CAD build for the part. Positions are in the model's coordinates, mm. Face numbers are marked on the shaded views. Round coordinates to 2 decimals unless told otherwise and drop trailing zeros. Loops run counter-clockwise (first coordinate to the right, second up) from the corner with the lowest first, then second, coordinate; pieces in that order, holes last. Notation, with made-up numbers: (59.5, 74) -> (113.5, 74) arc R19 cw to (113.5, 86) -> close; hole circle Ø10 at (10, 35). An arc over 180 degrees is marked (long way). Answer as CSV lines item,"result".
```python
from build123d import *

# Parameters (mm, degrees)
BOSS_EXTRUDE1_DEPTH = 600
CUT_EXTRUDE1_DEPTH  = 200
BOSS_EXTRUDE2_DEPTH = 20
FILLET1_R           = 5
SKETCH4_R           = 35
BOSS_EXTRUDE3_DEPTH = 20
BOSS_EXTRUDE4_START = 20
SKETCH5_R           = 35
BOSS_EXTRUDE4_DEPTH = 20
SKETCH6_R           = 10
CUT_EXTRUDE2_DEPTH  = 741.945342114
SKETCH7_R           = 25
BOSS_EXTRUDE5_DEPTH = 60
SKETCH9_R           = 20
CUT_EXTRUDE3_DEPTH  = 749.999332443
SKETCH10_R          = 7.841324839
BOSS_EXTRUDE6_DEPTH = 40
SKETCH11_R          = 3.5
BOSS_EXTRUDE7_DEPTH = 300
SKETCH12_R          = 4.427649499
BOSS_EXTRUDE8_DEPTH = 10


with BuildPart() as part:
    # Sketch1 → Boss-Extrude1 (new body)
    with BuildSketch(Plane.XY):
        Polygon((280, -110), (350, -40), (350, 110), (-350, 110), (-350, -110), align=None)
    extrude(amount=BOSS_EXTRUDE1_DEPTH)

    # Sketch2 → Cut-Extrude1 (cut)
    with BuildSketch(Plane(origin=(0, 110, 0), x_dir=(1, 0, 0), z_dir=(0, 1, 0))):
        Polygon((20.098635598, -30), (90.098635598, -300), (20.098635598, -570), (-320, -570), (-320, -30), align=None)
    extrude(amount=-CUT_EXTRUDE1_DEPTH, mode=Mode.SUBTRACT)

    # Sketch3 → Boss-Extrude2 (add)
    with BuildSketch(Plane(origin=(0, 110, 0), x_dir=(1, 0, 0), z_dir=(0, 1, 0))):
        Polygon((-330, -20), (-330, -580), (27.836654621, -580), (100.429247214, -300), (27.836654621, -20), align=None)
        Polygon((-320, -30), (-320, -570), (20.098635598, -570), (90.098635598, -300), (20.098635598, -30), align=None, mode=Mode.SUBTRACT)
    extrude(amount=BOSS_EXTRUDE2_DEPTH)

    # Fillet1
    fillet1_edges = [part.edges().sort_by_distance(p)[0] for p in [
        (-151.081672689, 130, 20),
        (-330, 130, 300),
        (-151.081672689, 130, 580),
        (64.132950917, 130, 440),
        (64.132950917, 130, 160),
        (-149.950682201, 130, 30),
        (-320, 130, 300),
        (-149.950682201, 130, 570),
        (55.098635598, 130, 435),
        (55.098635598, 130, 165),
    ]]
    fillet(fillet1_edges, radius=FILLET1_R - 0.0001)  # a hair under: the kernel refuses the full size

    # Sketch4 → Boss-Extrude3 (add)
    with BuildSketch(Plane.XY.offset(600)):
        with Locations(Location((270, 40, 0), (0, 0, 180))):
            Circle(SKETCH4_R)
    extrude(amount=BOSS_EXTRUDE3_DEPTH)

    # Sketch5 → Boss-Extrude4 (add)
    with BuildSketch(Plane(origin=(0, 0, 0), x_dir=(-1, 0, 0), z_dir=(0, 0, -1)).offset(BOSS_EXTRUDE4_START)):
        with Locations((-270, 40)):
            Circle(SKETCH5_R)
    extrude(amount=-BOSS_EXTRUDE4_DEPTH)

    # Sketch6 → Cut-Extrude2 (cut, through all)
    with BuildSketch(Plane.XY.offset(620)):
        with Locations((270, 40)):
            Circle(SKETCH6_R)
    extrude(amount=-CUT_EXTRUDE2_DEPTH, mode=Mode.SUBTRACT)

    # Sketch7 → Boss-Extrude5 (add)
    with BuildSketch(Plane(origin=(0, 110, 0), x_dir=(1, 0, 0), z_dir=(0, 1, 0))):
        with Locations(Location((177.752116484, -300, 0), (0, 0, 90))):
            Circle(SKETCH7_R)
    extrude(amount=BOSS_EXTRUDE5_DEPTH)

    # Sketch9 → Cut-Extrude3 (cut, through all)
    with BuildSketch(Plane.XY.offset(620)):
        with Locations((270, 40)):
            Circle(SKETCH9_R)
    extrude(amount=-CUT_EXTRUDE3_DEPTH, mode=Mode.SUBTRACT)

    # Sketch10 → Boss-Extrude6 (add)
    with BuildSketch(Plane(origin=(0, 110, 0), x_dir=(1, 0, 0), z_dir=(0, 1, 0))):
        with Locations(Location((-338.53526131, -590.113534013, 0), (0, 0, 90))):
            Circle(SKETCH10_R)
    extrude(amount=BOSS_EXTRUDE6_DEPTH)

    # Sketch11 → Boss-Extrude7 (add)
    with BuildSketch(Plane(origin=(0, 150, 0), x_dir=(1, 0, 0), z_dir=(0, 1, 0))):
        with Locations(Location((-338.53526131, -590.113534013, 0), (0, 0, 270))):
            Circle(SKETCH11_R)
    extrude(amount=BOSS_EXTRUDE7_DEPTH)

    # Sketch12 → Boss-Extrude8 (add)
    with BuildSketch(Plane(origin=(0, 450, 0), x_dir=(1, 0, 0), z_dir=(0, 1, 0))):
        with Locations(Location((-338.53526131, -590.113534013, 0), (0, 0, 270))):
            Circle(SKETCH12_R)
    extrude(amount=BOSS_EXTRUDE8_DEPTH)


solid = part.part
```
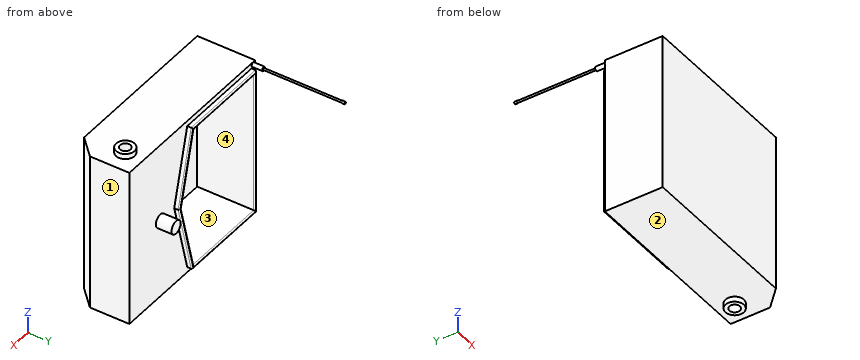
Q1. Probe L1, parallel to Z at x = -54.5, y = 88.5; L2, parallel to Y at x = 270, z = 288; L3, parallel to Y at x = 166, z = 276.5. List the from-to ranges inside material, lowest first. Write a range as [from, to].
Results:
L1,"[0, 30], [570, 600]"
L2,"[-110, 20], [60, 110]"
L3,"[-110, 110]"
Q2. Drop flat-ended pins along their axis: pin 1 Ø7.5 at (x, y) = (-211, 116) entering from +Z; pin 2 Ø6 at (x, z) = (-253.5, 118.5) entering from +Y; pin 3 Ø3 at (x, y) = (-172, 55) entering from +Z. Give the stop position or say it passes through.
Results:
pin 1,"z = 580"
pin 2,"y = -90"
pin 3,"z = 600"
Q3. Slice it at B-B, the plane x = 270. Give the cut face in (y, z), and give its area (3 significant figures).
Results:
outline,"(-110, 0) -> (5, 0) -> (5, -20) -> (20, -20) -> (20, 620) -> (5, 620) -> (5, 600) -> (-110, 600) -> close; (60, -20) -> (75, -20) -> (75, 0) -> (110, 0) -> (110, 600) -> (75, 600) -> (75, 620) -> (60, 620) -> close"
area,"109,000 mm2"
Q4. Two-plate mould, pull along X, no slides. Class the marked faces 1, 2, 3 and 4: pulls with the +X half, pulls with the -X half, needs draft (parallel to the pull), parting line crosses it, or undercut.
Results:
face 1,"pulls with the +X half"
face 2,"needs draft"
face 3,"undercut"
face 4,"undercut"
Q5. Slice it at C-C, the plane y = 100. Give the cut face in (x, z).
Results:
outline,"(-350, 0) -> (350, 0) -> (350, 600) -> (-350, 600) -> close; hole (-320, 30) -> (20.1, 30) -> (90.1, 300) -> (20.1, 570) -> (-320, 570) -> close"
Q6. Slice it at A-A, the plane y = 40. Give the cut face in (x, z).
Results:
outline,"(-350, 0) -> (235, 0) -> (235, -20) -> (250, -20) -> (250, 620) -> (235, 620) -> (235, 600) -> (-350, 600) -> close; (290, -20) -> (305, -20) -> (305, 0) -> (350, 0) -> (350, 600) -> (305, 600) -> (305, 620) -> (290, 620) -> close; hole (-320, 30) -> (20.1, 30) -> (90.1, 300) -> (20.1, 570) -> (-320, 570) -> close"
